Autodesk Inventor part; units mm, degrees
ref_plane "Work Plane5" through (0, 1.9, 0) normal (0, 1, 0) x (-1, 0, 0)
ref_plane "Work Plane9" through (0, -1, 0) normal (0, 1, 0) x (-1, 0, 0)
ref_plane "YZ Plane" through (0, 0, 0) normal (1, 0, 0) x (0, 1, 0)
sketch "Sketch11" plane through (0, 0, 0) normal (0, 1, 0) x (-1, 0, 0)
  circle A0 centre (0, 0) radius 1.9
  dimension "d86" = 3.8
sketch "Sketch12" plane through (0, 0, 0) normal (0, 1, 0) x (-1, 0, 0)
  circle A0 centre (0, 0) radius 1.3
  dimension "d87" = 2.6
ref_plane "Work Plane4" through (0, 2, 0) normal (0, 1, 0) x (-1, 0, 0)
ref_plane "Work Plane5" through (0, 1.9, 0) normal (0, 1, 0) x (-1, 0, 0)
extrude "Head" add sketch "Sketch11" along normal blind 2
chamfer "Chamfer3" distance 0.1 angle 60 1 edges at (1.9, 2, 0) measured on face at (-1.8938, 1.3333, -0.1529)
sketch "Sketch6" plane through (0, 1.9, 0) normal (0, 1, 0) x (1, 0, 0)
  line L0 (0, 0) -> (-1.9, 0) construction
  line L1 (0, 0) -> (-2, 0) construction
  line L2 (-2, 0) -> (-2, 0.2)
  line L3 (-2, 0) -> (-2, -0.2)
  line L4 (-2, -0.2) -> (-1.8894, -0.2)
  line L5 (-2, 0.2) -> (-1.8894, 0.2)
  line L6 (-1.8894, -0.2) -> (-1.8894, 0.2)
  circle A0 centre (0, 0) radius 1.9 construction
  dimension "d34" = 1.9
  dimension "d35" = 2
  dimension "d36" = 0.2
  dimension "d37" = 0.2
  dimension "d40" = 0.1106
  dimension "d75" = 3.8
extrude "Grip Knurling" [suppressed]
fillet "Fillet3" [suppressed]
pattern_circular "Circular Pattern1" [suppressed]
pattern_circular "Circular Pattern2" [suppressed]
sketch "Label" plane through (0, 2, 0) normal (0, 1, 0) x (-1, 0, 0)
  circle A0 centre (0, 0) radius 0.866
  circle A1 centre (0, 0) radius 1.7268
  dimension "shaftDiameter" = 2
  dimension "transitionDiameter" = 2.6
  dimension "d109" = 1.7321
feature "Bolt Designation" [suppressed]
sketch "Sketch2" plane through (0, 2, 0) normal (0, 1, 0) x (1, 0, 0)
  line L0 (0.75, -0.433) -> (0, -0.866)
  line L1 (0, -0.866) -> (-0.75, -0.433)
  line L2 (-0.75, -0.433) -> (-0.75, 0.433)
  line L3 (-0.75, 0.433) -> (0, 0.866)
  line L4 (0, 0.866) -> (0.75, 0.433)
  line L5 (0.75, 0.433) -> (0.75, -0.433)
  line L6 (-0.75, -0.433) -> (0.75, 0.433) construction
  point P0 (0, 0)
  point P1 (0, 0)
  dimension "d8" = 1.5
  dimension "d24" = 1.7321
  dimension "d85" = 0.866
extrude "HexagonSocket" [suppressed]
sketch "Sketch4" plane through (0, 2, 0) normal (0, 1, 0) x (1, 0, 0)
  circle A0 centre (0, 0) radius 0.866
  dimension "d25" = 1.7321
extrude "Socket_topTaper" cut sketch "Sketch4" against normal blind 0.116 draft -45
ref_plane "Work Plane8" through (0, 0.8, 0) normal (0, 1, 0) x (1, 0, 0)
sketch "Sketch10" plane through (0, 0.8, 0) normal (0, 1, 0) x (1, 0, 0)
  circle A0 centre (0, 0) radius 0.433
  dimension "d70" = 0.866
feature "Socket_bottomTaper" [suppressed]
extrude "Transition" add sketch "Sketch12" against normal blind 1
ref_plane "Work Plane9" through (0, -1, 0) normal (0, 1, 0) x (-1, 0, 0)
sketch "Sketch18" plane through (0, -1, 0) normal (0, -1, 0) x (1, 0, 0)
  circle A0 centre (0, 0) radius 1.3
extrude "Extruded Angle" add sketch "Sketch18" along normal blind 0.2 draft -56.31
sketch "Sketch19" plane through (0, -1.2, 0) normal (0, -1, 0) x (1, 0, 0)
  circle A0 centre (0, 0) radius 1
sketch "Sketch13" plane through (0, -1, 0) normal (0, -1, 0) x (1, 0, 0)
  circle A0 centre (0, 0) radius 1
  dimension "d92" = 2
extrude "Shaft" add sketch "Sketch13" along normal blind 19
fillet "Fillet4" radius 0.2 1 edges at (1.3, 0, 0)
chamfer "Chamfer4" distance 0.2 angle 45 1 edges at (-1, -20, 0)
thread "Thread1"
sketch "Sketch7" plane through (0, 0, 0) normal (0, 0, 1) x (1, 0, 0)
  line L0 (-1, 0.2) -> (1, 0.2) construction
  line L1 (-1, -20.4) -> (-0.7393, -20.5505)
  line L2 (-0.7393, -20.6495) -> (-1, -20.8)
  line L3 (-1, -20.8) -> (-1, -20.4)
  arc A0 (-0.7393, -20.6495) -> (-0.7393, -20.5505) centre (-0.7679, -20.6) ccw
  line L4 (-1, -19.8) -> (1, -19.8)
  point P0 (0, 0)
  point P1 (-0.8845, -20.6)
  point P2 (-0.6536, -20.6)
  dimension "d53" = 0.4
  dimension "d56" = 0.0571
  dimension "d124" = 0.6
  dimension "d125" = 0
feature "ModeledThreads" [suppressed]
extrude "Extrusion10" add sketch "Sketch19" against normal blind 1
equation "\"shaftDiameter\" = 2"
equation "\"transitionDiameter\" = 2.6"
equation "\"flangeCoupling_height\" = flangeCoupling_collarHeight + flangeCoupling_flangeHeight"
equation "\"headHeight\" = 2"
equation "\"headDiameter\" = 3.8"
equation "\"gap\" = 0.1"
equation "\"airgap\" = 0.4"
equation "\"wallgap\" = 2"
equation "\"printingLayerHeight\" = 0.2"
equation "\"driveMagnet_height\" = 5"
equation "\"halbachMagnet_height\" = 3"
equation "\"rotorBandBolt_diameter\" = 2"
equation "\"rotorBandBolt_headDiameter\" = 3.98"
equation "\"rotorBandBolt_headHeight\" = 2"
equation "\"rotorBandHexNut_sideToSide\" = 4"
equation "\"rotorBandHexNut_height\" = 1.2"
equation "\"rotorBandSquareNut_sideLength\" = 4"
equation "\"rotorBandSquareNut_height\" = 1.2"
equation "\"sensorMagnet_diameter\" = 5"
equation "\"sensorMagnet_height\" = 2.66667"
equation "\"sensorMagnet_ringRadius\" = 0.5 * driveMagnet_centerSpacingRadius + 2 * wallgap"
equation "\"rotorRadius\" = 2 * gap + driveMagnet_centerSpacingRadius + driveMagnet_length + wallgap"
equation "\"rotor_mountingLipHeight\" = 0.5 * statorThickness"
equation "\"flangeBearing_innerDiameter\" = shaftDiameter"
equation "\"flangeBearing_outerDiameter\" = 16"
equation "\"flangeBearing_flangeDiameter\" = 18"
equation "\"flangeBearing_height\" = 5"
equation "\"flangeBearing_flangeHeight\" = 1"
equation "\"magnetWire_outerDiameter\" = 0.8128"
equation "\"coilThickness\" = 12"
equation "\"statorThickness\" = coilThickness + 2 * wallgap"
equation "\"rotorBandThickness\" = wallgap + rotorBandBolt_headHeight + gap"
equation "\"flangeCoupling_innerDiameter\" = shaftDiameter"
equation "\"flangeCoupling_collarOuterDiameter\" = 16"
equation "\"flangeCoupling_flangeDiameter\" = 32"
equation "\"flangeCoupling_flangeHeight\" = 3.1"
equation "\"flangeCoupling_mountHoleDiameter\" = 3.9"
equation "\"flangeCoupling_mountHoleEdgeToEdge\" = 2.05"
equation "\"statorRadius\" = driveMagnet_length + driveMagnet_centerSpacingRadius + 2 * gap"
equation "\"statorMountBolt_diameter\" = 4"
equation "\"statorMountBolt_headDiameter\" = 7"
equation "\"statorMountBolt_headHeight\" = 4"
equation "\"statorMountBolt_shaftLength\" = coilThickness + flangeCoupling_flangeHeight + wallgap"
equation "\"statorMountHexNut_sideToSide\" = 8"
equation "\"statorMountHexNut_height\" = 4"
equation "\"coil_percentCoverage\" = 0.6"
equation "\"statorSpokeDegrees\" = 4deg"
equation "\"statorCoilBolt_diameter\" = 2"
equation "\"statorCoilBolt_headDiameter\" = 3.98"
equation "\"statorCoilBolt_headHeight\" = 2"
equation "\"statorCoilBolt_shaftLength\" = coilThickness"
equation "\"statorCoilHexNut_sideToSide\" = 4"
equation "\"statorCoilHexNut_height\" = 1.2"
equation "\"circuitBoard_height\" = 1.6"
equation "\"hallEffectSensor_height\" = 1.1"
equation "\"hallEffectSensor_length\" = 3"
equation "\"hallEffectSensor_width\" = 1.6"
equation "\"hallEffectSensor_pinLength\" = 0.6"
equation "\"circuitboardMountBolt_diameter\" = 2"
equation "\"circuitboardMountBolt_headDiameter\" = 3.98"
equation "\"circuitboardMountBolt_headHeight\" = 2"
equation "\"circuitboardMountBolt_shaftLength\" = coilThickness"
equation "\"circuitboardMountHexNut_sideToSide\" = 4"
equation "\"circuitboardMountHexNut_height\" = 1.2"
equation "\"statorShellBolt_diameter\" = 3"
equation "\"statorShellBolt_headDiameter\" = 5.68"
equation "\"statorShellBolt_headHeight\" = 3"
equation "\"statorShellBolt_shaftLength\" = statorThickness - statorShellBolt_countersinkDepth"
equation "\"statorShellHexNut_sideToSide\" = 5.3"
equation "\"statorShellHexNut_height\" = 2.3"
equation "\"threadPitch\" = 0.4"
equation "\"socketSize\" = 1.5"
equation "\"chamferSize\" = 0.2"
equation "\"keyEngagementDepth\" = 1"
equation "\"transitionLength\" = 1"
equation "\"textSize\" = 0.95"
properties part number "M2" material "Steel, Galvanized"
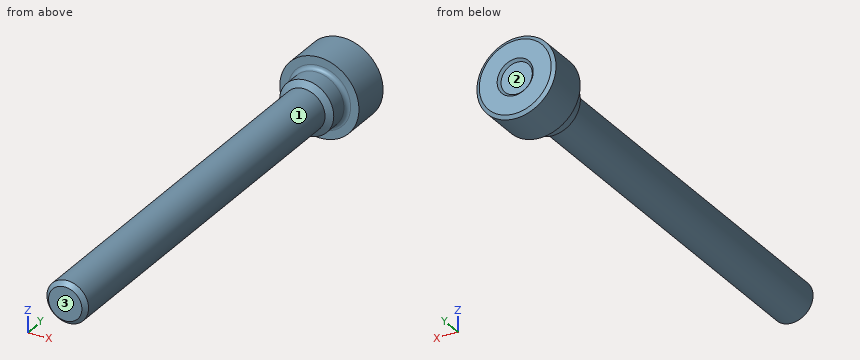
Check sheet for the modelled part. Datum: model origin and axes. Units: mm. Face numbers are marked on the shaded views. A direction names the side the tool comes from. Give positions to 0.01 mm unless a question says otherwise; leave off trailing zeros. Loops run counter-clockwise (first coordinate to the right, second up) from the corner with the lowest first, then second, coordinate; pieces in that order, holes last. Notation, with made-up numbers: M 20,26 L 71,26 A26 cw 71,51 Z; hole C 9,28.5 d7. An arc over 180 degrees is marked long. Use a Markdown table: item, result. Add a question column.
Q1. Sectioned sample at B-B, the plane z = 0. Record the cut outline in (x, y), then the cut area to 3 significant figures.
Q2. Tool access check on the marked faces 1, 2 and 3. Record the directions out of +Z, -Z, +X, -X, +Y, -Y that give a thin tool (end or side, any length) a straight path to the whole face; none if there is none.
Q3. Go/stop test with flat-tipped pins: pin 1 (1.5 mm diameter, centred on x = 0.5, y = -2, fed in from +Z); pin 2 (0.8 mm diameter, centred on x = 0.5, z = -0.5, fed in from +Y). Record where each tip stops, or that it passes through.
Q4. Scan lines: line 1 along Z through (x, y) = (-0.1, -2.5); line 2 along Y through (x, z) = (0, -1.65); line 3 along Y through (x, z) = (0.75, -0.15). Record each from-to range of solid material in increasing order. Write a range as [from, to].
Q5. Sectioned sample at A-A, the plane x = 0. Record the cut outline in (y, z).
Q6. Sectioned sample at C-C, the plane y = -18.5. Record the cut outline in (x, z).
Verdict:
| question | item | result |
|---|---|---|
| 1 | outline | M -1.9,0 L -1.5,0 A0.2 cw -1.3,-0.2 L -1.3,-1 L -1,-1.2 L -1,-19.8 L -0.8,-20 L 0.8,-20 L 1,-19.8 L 1,-1.2 L 1.3,-1 L 1.3,-0.2 A0.2 cw 1.5,0 L 1.9,0 L 1.9,1.9 L 1.73,2 L 0.87,2 L 0.75,1.88 L -0.75,1.88 L -0.87,2 L -1.73,2 L -1.9,1.9 Z |
| 1 | area | 48.0 mm^2 |
| 2 | face 1 | -Y |
| 2 | face 2 | +Y |
| 2 | face 3 | +Z, -Z, +X, -X, -Y |
| 3 | pin 1 | z = 1 |
| 3 | pin 2 | y = 2 |
| 4 | line 1 | [-0.99, 0.99] |
| 4 | line 2 | [0, 2] |
| 4 | line 3 | [-20, 1.9] |
| 5 | outline | M -20,-0.8 L -19.8,-1 L -1.2,-1 L -1,-1.3 L -0.2,-1.3 A0.2 cw 0,-1.5 L 0,-1.9 L 1.9,-1.9 L 2,-1.73 L 2,-0.87 L 1.88,-0.75 L 1.88,0.75 L 2,0.87 L 2,1.73 L 1.9,1.9 L 0,1.9 L 0,1.5 A0.2 cw -0.2,1.3 L -1,1.3 L -1.2,1 L -19.8,1 L -20,0.8 Z |
| 6 | outline | C 0,0 d2 |
